Autodesk Inventor part; units mm, degrees
ref_plane "YZ Plane" through (0, 0, 0) normal (1, 0, 0) x (0, 1, 0)
ref_plane "XZ Plane" through (0, 0, 0) normal (0, 1, 0) x (-1, 0, 0)
ref_plane "XY Plane" through (0, 0, 0) normal (0, 0, 1) x (1, 0, 0)
sketch "Sketch1" plane through (0, 0, 0) normal (0, 0, 1) x (1, 0, 0)
  line L0 (0, 0) -> (-70, 0)
  line L1 (0, 0) -> (0, -10)
  line L2 (0, -10) -> (-26.6667, -10)
  line L3 (-26.6667, -10) -> (-70, -20)
  line L4 (-70, -20) -> (-70, 0)
  circle A0 centre (-5, -5) radius 2.5
  dimension "d0" = 70
  dimension "d1" = 5
  dimension "d2" = 10
  dimension "d3" = 5
  dimension "d4" = 5
  dimension "d5" = 20
extrude "Extrusion1" add sketch "Sketch1" along normal blind 18
fillet "Fillet4" radius 4 1 edges at (-26.6667, -10, 9)
fillet "Fillet5" radius 5 2 edges at (0, 0, 9) (0, -10, 9)
sketch "Sketch4" plane through (-70, -20, 0) normal (0.2249, -0.9744, 0) x (0.9744, 0.2249, 0)
  circle A0 centre (6, 9) radius 4
  line L0 (44.0167, 18) -> (44.0167, 0)
  line L1 (0, 18) -> (44.0167, 18)
  line L2 (0, 0) -> (0, 18)
  line L3 (0, 0) -> (44.0167, 0)
  point P0 (72.7046, 0)
  dimension "d24" = 8
  dimension "d25" = 6
  dimension "d26" = 9
extrude "Extrusion4" add sketch "Sketch4" along normal blind 5 contours A0
fillet "Fillet6" radius 1 1 edges at (-66.9269, -24.4222, 9)
sketch "Sketch5" plane through (-70, 0, 0) normal (0, 1, 0) x (1, 0, 0)
  line L0 (15, 0) -> (30, 0)
  line L1 (30, 0) -> (30, -11.5)
  line L2 (30, -11.5) -> (15, -11.5)
  line L3 (15, -11.5) -> (15, 0)
  line L4 (65, -18) -> (0, -18)
  line L5 (0, 0) -> (0, -18)
  line L6 (65, 0) -> (0, 0)
  point P0 (70, 0)
  point P1 (0, -3.5)
  dimension "d31" = 15
  dimension "d33" = 6.5
  dimension "d34" = 15
extrude "Extrusion5" add sketch "Sketch5" along normal blind 40
sketch "Sketch6" plane through (-40, 0, 11.5) normal (0, 0, 1) x (1, 0, 0)
  circle A0 centre (-5, 35) radius 3
  line L0 (-15, 40) -> (0, 40)
  line L1 (0, 0) -> (0, 40)
  point P0 (40, 0)
  dimension "d37" = 6
  dimension "d38" = 5
  dimension "d39" = 5
extrude "Extrusion6" cut sketch "Sketch6" against normal up to next
sketch "Sketch7" plane through (-55, 0, 0) normal (-1, 0, 0) x (0, 0, 1)
  line L0 (0, 40) -> (6.5, 40)
  line L1 (0, 20) -> (0, 40)
  line L2 (6.5, 40) -> (6.5, 20)
  line L3 (6.5, 20) -> (0, 20)
  line L4 (0, 0) -> (0, 40)
  line L5 (11.5, 0) -> (11.5, 40)
  line L6 (0, 40) -> (11.5, 40)
  dimension "d42" = 5
  dimension "d44" = 20
extrude "Extrusion7" cut sketch "Sketch7" against normal up to next
fillet "Fillet8" radius 5 2 edges at (-40, 40, 9) (-55, 40, 9)
fillet "Fillet9" radius 2 3 edges at (-55, 0, 5.75) (-47.5, 0, 11.5) (-40, 0, 5.75)
fillet "Fillet10" radius 2 1 edges at (-70, -20, 9)
properties part number "Swinging_connection" material "Wood (Cherry)"
Source: CAD feature listing. Evaluate the final solid. Frame: model axes, mm. A direction names the side the tool comes from. Coordinates: 2 decimals unless noted, no trailing zeros. Loops run counter-clockwise (first coordinate to the right, second up) from the corner with the lowest first, then second, coordinate; pieces in that order, holes last. Notation, with made-up numbers: (-7.75, -26) -> (23.25, -26) arc R17 cw to (23.25, -15) -> close; hole circle Ø6 at (62.25, 4). An arc over 180 degrees is marked (long way). One line per item, written item: value. Start each with the question number.
Q1. Section query A-A, the plane x = -6.5. Return the cut outline in (y, z).
Q2. Section query C-C, the plane x = -41. Return the cut outline in (y, z), and give its area (3 significant figures).
Q3. Section query D-D, the plane y = 6. Return the cut outline in (x, z).
Q4. Contact query for flat-ended pins moving along their axis: P1, Ø10, axis at x = -31, z = 2.5, coming from the -Y side; P2, Ø12, axis at x = -49.5, y = 22.5, coming from the +Z side; P3, Ø6, axis at x = -5, y = -5, coming from the +Z side; P4, Ø3.5, axis at y = 15, z = 5, coming from the -X side. Output: stop coordinate, or through.
Q5. Line query: line 1 along Y through (x, z) = (-5, 3.5); line 2 along X through (y, z) = (19.5, 6.5); line 3 along Z through (x, y) = (-54, 15). Output: solid intervals per line, ascending.
Q6. Set-up query: faces 1 (the face through (-15, -10, 9)), 2 (the face through (-48, 20, 3)), 3 (the face through (-55, 15, 7)), 4 (the face through (-47, 21, 11.5)). Return all of +Z, -Z, +X, -X, +Y, -Y with unobstructed straight access to the full face (end or side cutting, diameter ignored); none if empty.
Q7. Mould query, pull axis Y, two halves, no side actions, for faces 5 (the face through (-40, 15, 7)), 6 (the face through (-47.21, 37.03, 9.04)), 7 (the face through (-69.26, -19.04, 14.53)). Classes: pulls with the +Y half, pulls with the -Y half, needs draft (parallel to the pull), parting line crosses it, or undercut.
Results:
1. outline: (-10, 0) -> (-7, 0) -> (-7, 18) -> (-10, 18) -> close; (-3, 0) -> (0, 0) -> (0, 18) -> (-3, 18) -> close
2. outline: (-13.31, 0) -> (20, 0) -> (20, 6.5) -> (38, 6.5) -> (38, 11.5) -> (2, 11.5) arc R2 cw to (0, 13.5) -> (0, 18) -> (-13.31, 18) -> close
2. area: 560 mm^2
3. outline: (-55, 0) -> (-40, 0) -> (-40, 11.5) -> (-55, 11.5) -> close
4. P1: y = -12.15
4. P2: z = 11.5
4. P3: z = 18
4. P4: x = -55
5. line 1: -10 to -7.5, -2.5 to 0
5. line 2: -55 to -40
5. line 3: 0 to 11.5
6. face 1: +Z, -Z, +X, -Y
6. face 2: -Z, +X, -X, +Y
6. face 3: +Z, -Z, -X, +Y
6. face 4: +Z, +X, -X, +Y
7. face 5: needs draft
7. face 6: undercut
7. face 7: pulls with the -Y half
